For this review, take the finished solid that the model builds, in its own axes (mm). A direction names the side the tool comes from. Give positions to 0.01 mm unless a question says otherwise; leave off trailing zeros. Order: outer loops, then holes, each group sorted by start corner. A loop starts at its lowest first (then second) coordinate and runs counter-clockwise, first axis right, second up.
Item 1: Consider section A-A (z = -276). Give the boundary of the cut face in (x, y).
Item 2: Consider section D-D (x = -22). Give the boundary of the cut face in (y, z).
Item 3: Machinability: for faces 1 (the flat face through (200, -235, -231)), 2 (the flat face through (280, -179, -198)), 3 (the flat face through (300, -170, -178)), 4 (the flat face through (-204, -250, -128)), 5 (the flat face through (-287, -130, -231)), which of the approach directions +Z, -Z, +X, -X, +Y, -Y give a long, thin tool a straight path to every point of the face, cutting with its end or side? Answer none if there is none.
Item 4: Consider section B-B (x = -218). Give the boundary of the cut face in (y, z).
Item 5: For P1, Ø12, axis at x = -136, y = -2, coming from the -Z side, flat-tipped, find the tip position at first contact; note if it passes through.
Item 6: For probe 1 along X at (y, z) = (167.5, -26); probe 2 along Z at (x, y) = (-232, -216.5); probe 3 along Z at (x, y) = (-97, 207.5), list the stretches that pass through material, from the lowest coordinate up.
Item 7: The part is to be moulded in two halves that separate along Z. For faces 6 (the flat face through (204, 250, -128)), 7 (the flat face through (241, 181, -390)), 8 (the flat face through (-4, 4, 50)), 9 (the flat face through (-249, -189, -400)), say which applies: released by +Z, released by -Z, zero draft, split by the parting line, or undercut.
Item 8: Consider section C-C (y = -183.5). Give the boundary of the cut face in (x, z), plus the area to 3 significant figures.
Autodesk Inventor part; units mm, degrees
ref_plane "YZ Plane" through (0, 0, 0) normal (1, 0, 0) x (0, 1, 0)
ref_plane "XZ Plane" through (0, 0, 0) normal (0, 1, 0) x (-1, 0, 0)
ref_plane "XY Plane" through (0, 0, 0) normal (0, 0, 1) x (1, 0, 0)
sketch "Boceto1" plane through (0, 0, 0) normal (0, 0, 1) x (1, 0, 0)
  line L0 (-300, -250) -> (300, -250)
  line L1 (300, -250) -> (300, 250)
  line L2 (300, 250) -> (-300, 250)
  line L3 (-300, 250) -> (-300, -250)
  line L4 (-300, -250) -> (300, 250) construction
  line L5 (300, -250) -> (-300, 250) construction
  line L6 (-300, 250) -> (-200, 250)
  line L7 (-200, 250) -> (-200, 230)
  line L8 (-280, 130) -> (-300, 130)
  line L9 (-300, 130) -> (-300, 250)
  line L10 (-300, 130) -> (-280, 130)
  line L11 (-280, 130) -> (-280, 230)
  line L12 (-280, 230) -> (-200, 230)
  line L13 (0, 0) -> (0, 50)
  line L14 (0, 0) -> (-60, 0)
  line L15 (-300, 250) -> (300, 250)
  line L16 (300, 250) -> (300, -250)
  line L17 (-300, -250) -> (300, 250) construction
  line L18 (300, 250) -> (200, 250)
  line L19 (200, 250) -> (200, 230)
  line L20 (300, 130) -> (300, 250)
  line L21 (280, 130) -> (280, 230)
  line L22 (280, 230) -> (200, 230)
  line L23 (280, 130) -> (300, 130)
  line L24 (300, -250) -> (-300, -250)
  line L25 (-300, -250) -> (-300, 250)
  line L26 (300, 250) -> (-300, -250) construction
  line L27 (-300, -250) -> (-200, -250)
  line L28 (-200, -250) -> (-200, -230)
  line L29 (-280, -130) -> (-300, -130)
  line L30 (-300, -130) -> (-300, -250)
  line L31 (-300, -130) -> (-280, -130)
  line L32 (-280, -130) -> (-280, -230)
  line L33 (-280, -230) -> (-200, -230)
  line L34 (-300, -250) -> (300, -250)
  line L35 (300, -250) -> (200, -250)
  line L36 (200, -250) -> (200, -230)
  line L37 (300, -130) -> (300, -250)
  line L38 (280, -130) -> (280, -230)
  line L39 (280, -230) -> (200, -230)
  line L40 (280, -130) -> (300, -130)
  point P0 (-300, 130)
  point P1 (-300, -130)
  point P2 (-200, -250)
  point P3 (200, -250)
  point P4 (300, -130)
  point P5 (300, 130)
  point P6 (200, 250)
  point P7 (-200, 250)
  dimension "d0" = 600
  dimension "d1" = 500
  dimension "d4" = 20
  dimension "d5" = 100
  dimension "d6" = 60
  dimension "d13" = 20
extrude "Extrusión1" add sketch "Boceto1" along normal blind 50 contours L28 L33 L32 L29 L3 L8 L11 L12 L7 L2 L19 L22 L21 L23 L1 L40 L38 L39 L36 L0
extrude "Extrusión2" add sketch "Boceto1" along normal blind 50 and the other way blind 390 contours L3 L29 L32 L33 L28 L0 | L36 L39 L38 L40 L1 L0 | L3 L2 L7 L12 L11 L8 | L23 L21 L22 L19 L2 L1
sketch "Boceto2" plane through (0, 0, -390) normal (0, 0, -1) x (-1, 0, 0)
  line L0 (280, 230) -> (280, 130)
  line L1 (200, 230) -> (280, 230)
  line L2 (200, 250) -> (200, 230)
  line L3 (-200, 250) -> (200, 250)
  line L4 (-200, 230) -> (-200, 250)
  line L5 (-280, 230) -> (-200, 230)
  line L6 (-280, 130) -> (-280, 230)
  line L7 (-300, 130) -> (-280, 130)
  line L8 (-300, -130) -> (-300, 130)
  line L9 (-280, -130) -> (-300, -130)
  line L10 (-280, -230) -> (-280, -130)
  line L11 (-200, -230) -> (-280, -230)
  line L12 (-200, -250) -> (-200, -230)
  line L13 (200, -250) -> (-200, -250)
  line L14 (200, -230) -> (200, -250)
  line L15 (280, -230) -> (200, -230)
  line L16 (280, -130) -> (280, -230)
  line L17 (300, -130) -> (280, -130)
  line L18 (300, 130) -> (300, -130)
  line L19 (280, 130) -> (300, 130)
  line L20 (300, 250) -> (300, -250)
  line L21 (300, -250) -> (200, -250)
  line L22 (200, -250) -> (200, -130)
  line L23 (200, -130) -> (300, -130)
  line L24 (300, -130) -> (300, -250)
  line L25 (-300, 250) -> (-200, 250)
  line L26 (-200, 250) -> (-200, 130)
  line L27 (-200, 130) -> (-300, 130)
  line L28 (-300, 130) -> (-300, 250)
  line L29 (300, 250) -> (200, 250)
  line L30 (200, 250) -> (200, 130)
  line L31 (200, 130) -> (300, 130)
  line L32 (300, 130) -> (300, 250)
  line L33 (-300, -250) -> (-200, -250)
  line L34 (-200, -250) -> (-200, -130)
  line L35 (-200, -130) -> (-300, -130)
  line L36 (-300, -130) -> (-300, -250)
  point P0 (0, 0)
extrude "Extrusión3" add sketch "Boceto2" along normal blind 10 contours L1 L2 L29 L20 L19 L0 | L0 L31 L30 L1 | L20 L21 L14 L15 L16 L17 | L4 L5 L6 L7 L28 L25 | L16 L15 L22 L23 | L26 L27 L6 L5 | L33 L36 L9 L10 L11 L12 | L11 L10 L35 L34
properties part number "MESA_TALADRADO"
Resolved:
1. outline: (-300, -250) - (-200, -250) - (-200, -230) - (-280, -230) - (-280, -130) - (-300, -130) - close; (-300, 130) - (-280, 130) - (-280, 230) - (-200, 230) - (-200, 250) - (-300, 250) - close; (200, -250) - (300, -250) - (300, -130) - (280, -130) - (280, -230) - (200, -230) - close; (200, 230) - (280, 230) - (280, 130) - (300, 130) - (300, 250) - (200, 250) - close
2. outline: (-250, 0) - (250, 0) - (250, 50) - (-250, 50) - close
3. face 1: -Z, +Y, -Y
3. face 2: none
3. face 3: +Z, -Z, +X, +Y, -Y
3. face 4: +Z, -Z, +X, -X, -Y
3. face 5: -Z, +X, -X
4. outline: (-250, -400) - (-130, -400) - (-130, -390) - (-230, -390) - (-230, 0) - (230, 0) - (230, -390) - (130, -390) - (130, -400) - (250, -400) - (250, 50) - (-250, 50) - close
5. P1: stops at z = 0
6. probe 1: x = -300 to -280, 280 to 300
6. probe 2: z = -400 to -390, 0 to 50
6. probe 3: z = 0 to 50
7. face 6: zero draft
7. face 7: undercut
7. face 8: released by +Z
7. face 9: released by -Z
8. outline: (-300, -400) - (-200, -400) - (-200, -390) - (-280, -390) - (-280, 0) - (280, 0) - (280, -390) - (200, -390) - (200, -400) - (300, -400) - (300, 50) - (-300, 50) - close
8. area: 47,600 mm2
